Check sheet for the modelled part. Datum: model origin and axes. Units: mm. A direction names the side the tool comes from. Round coordinates to 2 decimals unless told otherwise and drop trailing zeros. Write each loop counter-clockwise with the first axis right and the second up, starting at its lowest first coordinate (ties: lowest second). Pieces come first, ordered by that corner, then holes. Notation, with made-up numbers: (18.25, -27.75) -> (68.25, -27.75) arc R14 ccw to (68.25, -13.75) -> close; hole circle Ø8 at (35.25, 54). An arc over 180 degrees is marked (long way). One line per item, written item: value.
from build123d import *

# Parameters (mm, degrees)
SKETCH1_W           = 10.287
SKETCH1_H           = 20.701
SKETCH1_R           = 2.1
SKETCH1_W_2         = 20.701
SKETCH1_H_2         = 10.287
SKETCH1_H_3         = 1.524
SKETCH1_W_3         = 1.524
BOSS_EXTRUDE1_DEPTH = 5.08
BOSS_EXTRUDE2_DEPTH = 5.08
FILLET1_R           = 0.1905


with BuildPart() as part:
    # Sketch1 → Boss-Extrude1 (new body)
    # profile 1 of 12: a face of its own
    with BuildSketch(Plane(origin=(0, 0, 0), x_dir=(1, 0, 0), z_dir=(0, 1, 0))):
        Polygon((13.335, 1.524), (13.335, 0), (35.56, 0), (35.56, 13.335), (13.335, 13.335), (13.335, 11.811), (34.036, 11.811), (34.036, 1.524), align=None)
    # profile 2 of 12: a face of its own
    with BuildSketch(Plane(origin=(0, 0, 0), x_dir=(1, 0, 0), z_dir=(0, 1, 0))):
        Polygon((0, 35.56), (0, 13.335), (1.524, 13.335), (1.524, 34.036), (11.811, 34.036), (11.811, 13.335), (13.335, 13.335), (13.335, 35.56), align=None)
    # profile 3 of 12: a face of its own
    with BuildSketch(Plane(origin=(0, 0, 0), x_dir=(1, 0, 0), z_dir=(0, 1, 0))):
        with Locations((6.6675, 23.6855)):
            Rectangle(SKETCH1_W, SKETCH1_H)
        with Locations(Location((6.6675, 24.4475, 0), (0, 0, 270))):
            Circle(SKETCH1_R, mode=Mode.SUBTRACT)
    # profile 4 of 12: a face of its own
    with BuildSketch(Plane(origin=(0, 0, 0), x_dir=(1, 0, 0), z_dir=(0, 1, 0))):
        Polygon((11.811, 11.811), (1.524, 1.524), (11.811, 1.524), align=None)
    # profile 5 of 12: a face of its own
    with BuildSketch(Plane(origin=(0, 0, 0), x_dir=(1, 0, 0), z_dir=(0, 1, 0))):
        Polygon((1.524, 11.811), (1.524, 1.524), (11.811, 11.811), align=None)
    # profile 6 of 12: a face of its own
    with BuildSketch(Plane(origin=(0, 0, 0), x_dir=(1, 0, 0), z_dir=(0, 1, 0))):
        with Locations((23.6855, 6.6675)):
            Rectangle(SKETCH1_W_2, SKETCH1_H_2)
        with Locations(Location((24.4475, 6.6675, 0), (0, 0, 270))):
            Circle(SKETCH1_R, mode=Mode.SUBTRACT)
    # profile 7 of 12: a face of its own
    with BuildSketch(Plane(origin=(0, 0, 0), x_dir=(1, 0, 0), z_dir=(0, 1, 0))):
        Polygon((11.811, 13.335), (11.811, 11.811), (13.335, 13.335), align=None)
    # profile 8 of 12: a face of its own
    with BuildSketch(Plane(origin=(0, 0, 0), x_dir=(1, 0, 0), z_dir=(0, 1, 0))):
        Polygon((13.335, 13.335), (11.811, 11.811), (13.335, 11.811), align=None)
    # profile 9 of 12: a face of its own
    with BuildSketch(Plane(origin=(0, 0, 0), x_dir=(1, 0, 0), z_dir=(0, 1, 0))):
        with Locations((6.6675, 12.573)):
            Rectangle(SKETCH1_W, SKETCH1_H_3)
    # profile 10 of 12: a face of its own
    with BuildSketch(Plane(origin=(0, 0, 0), x_dir=(1, 0, 0), z_dir=(0, 1, 0))):
        with Locations((12.573, 6.6675)):
            Rectangle(SKETCH1_W_3, SKETCH1_H_2)
    # profile 11 of 12: a face of its own
    with BuildSketch(Plane(origin=(0, 0, 0), x_dir=(1, 0, 0), z_dir=(0, 1, 0))):
        Polygon((0, 13.335), (0, 0), (1.524, 1.524), (1.524, 11.811), (1.524, 13.335), align=None)
    # profile 12 of 12: a face of its own
    with BuildSketch(Plane(origin=(0, 0, 0), x_dir=(1, 0, 0), z_dir=(0, 1, 0))):
        Polygon((1.524, 1.524), (0, 0), (13.335, 0), (13.335, 1.524), (11.811, 1.524), align=None)
    extrude(amount=BOSS_EXTRUDE1_DEPTH)

    # Sketch1_3 → Boss-Extrude2 (add)
    with BuildSketch(Plane(origin=(0, 0, 0), x_dir=(1, 0, 0), z_dir=(0, 1, 0))):
        Polygon((13.335, 1.524), (13.335, 0), (35.56, 0), (35.56, 13.335), (13.335, 13.335), (13.335, 11.811), (34.036, 11.811), (34.036, 1.524), align=None)
        Polygon((1.524, 1.524), (0, 0), (13.335, 0), (13.335, 1.524), (11.811, 1.524), align=None)
        Polygon((0, 13.335), (0, 0), (1.524, 1.524), (1.524, 11.811), (1.524, 13.335), align=None)
        Polygon((0, 35.56), (0, 13.335), (1.524, 13.335), (1.524, 34.036), (11.811, 34.036), (11.811, 13.335), (13.335, 13.335), (13.335, 35.56), align=None)
        Polygon((13.335, 13.335), (11.811, 11.811), (13.335, 11.811), align=None)
        Polygon((11.811, 13.335), (11.811, 11.811), (13.335, 13.335), align=None)
    extrude(amount=-BOSS_EXTRUDE2_DEPTH)

    # Fillet1
    fillet1_edges = [part.edges().sort_by_distance(p)[0] for p in [
        (13.335, 5.08, -24.4475),
        (35.56, 0, -13.335),
        (6.6675, 5.08, -35.56),
        (35.56, 0, 0),
        (0, 0, 0),
        (0, 0, -35.56),
        (13.335, 0, -35.56),
        (13.335, 0, -13.335),
        (0, 5.08, -17.78),
        (17.78, 5.08, 0),
        (13.335, -5.08, -24.4475),
        (35.56, -5.08, -6.6675),
        (17.78, -5.08, 0),
        (1.524, -5.08, -17.78),
        (35.56, 5.08, -6.6675),
        (22.9235, -5.08, -11.811),
        (6.6675, -5.08, -34.036),
        (17.78, -5.08, -1.524),
        (34.036, -5.08, -6.6675),
        (11.811, -5.08, -22.9235),
        (6.6675, -5.08, -35.56),
        (24.4475, -5.08, -13.335),
        (0, -5.08, -17.78),
        (24.4475, 5.08, -8.7675),
        (6.6675, 5.08, -26.5475),
        (24.4475, 5.08, -13.335),
    ]]
    fillet(fillet1_edges, radius=FILLET1_R)


solid = part.part
Item 1: Depth check by flat-ended pin: P1, Ø2.5, axis at y = -2, z = -17, coming from the +X side (3 decimals); P2, Ø5, axis at x = 7, z = -9, coming from the -Y side; P3, Ø2.5, axis at x = 24.45, z = -6.67, coming from the +Y side; P4, Ø5.5, axis at x = 20, y = -3.5, coming from the -Z side (3 decimals). Enter the tip coordinate at first touch or a pass-through.
Answer:
P1: stops at x = 13.335
P2: stops at y = 0
P3: passes through
P4: stops at z = -13.335
Item 2: Thickness scan on line 1 (X direction, y = -1.25, z = -16.5) (3 decimals); line 2 (Z direction, x = 21, y = -1.25) (3 decimals); line 3 (X direction, y = -3.5, z = -12). Record the ranges inside material, lowest first.
Answer:
line 1: x = 0 to 1.524, 11.811 to 13.335
line 2: z = -13.335 to -11.811, -1.524 to 0
line 3: x = 0 to 1.52, 11.81 to 35.56
Item 3: Sectioned sample at D-D on x = 10.5. Enter the section's corners in (y, z).
Answer:
outline: (-5.08, -35.37) arc R0.19 ccw to (-4.89, -35.56) -> (4.89, -35.56) arc R0.19 ccw to (5.08, -35.37) -> (5.08, -0.19) arc R0.19 ccw to (4.89, 0) -> (-4.89, 0) arc R0.19 ccw to (-5.08, -0.19) -> (-5.08, -1.33) arc R0.19 ccw to (-4.89, -1.52) -> (0, -1.52) -> (0, -34.04) -> (-4.89, -34.04) arc R0.19 ccw to (-5.08, -34.23) -> close
Item 4: Sectioned sample at B-B on y = 0.75. Count the separate pieces of the cut face and the enclosed holes in it, and give its area (3 significant figures).
Answer:
separate pieces: 1
enclosed holes: 2
area: 743 mm^2
Item 5: Tool access check on faces 5 (the flat face through (12.5, -5.08, -14)), 6 (the flat face through (13.335, 0, -24)), 7 (the flat face through (34.036, -2, -7)). Record the directions out of +Z, -Z, +X, -X, +Y, -Y that give a thin tool (end or side, any length) a straight path to the whole face; none if there is none.
Answer:
face 5: +Z, -Z, +X, -X, -Y
face 6: -Z, +X, +Y, -Y
face 7: -Y
Item 6: Mould release check, pull along Z, two halves, no side actions. Record for faces 1 (the flat face through (14, 5.08, -10)), 2 (the flat face through (7, 0, -35.56)), 3 (the flat face through (10, 0, -14)), 4 (the flat face through (23, -2, -11.811)): pulls with the +Z half, pulls with the -Z half, needs draft (parallel to the pull), parting line crosses it, or undercut.
Answer:
face 1: needs draft
face 2: pulls with the -Z half
face 3: undercut
face 4: undercut
